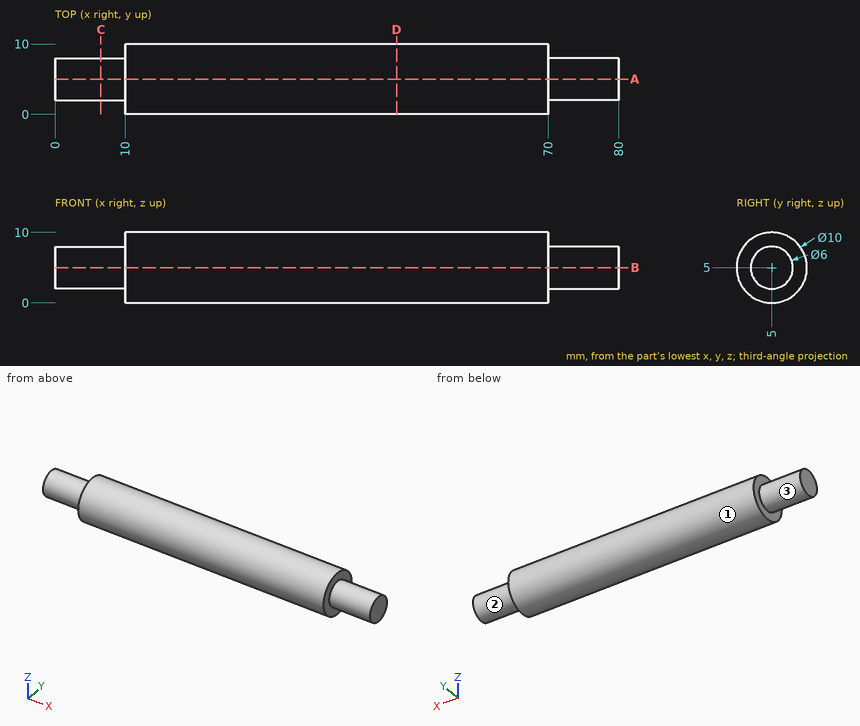
Source: three-view drawing plus pictorial views. Frame: mm from the lowest corner of the part. A direction names the side the tool comes from. Coordinates: 2 decimals unless noted, no trailing zeros. Order: outer loops, then holes, each group sorted by start corner. A loop starts at its lowest first (then second) coordinate and runs counter-clockwise, first axis right, second up. Notation, with made-up numbers: M 40.25,-10 L 61.25,-10 A33 cw 61.25,29 Z; hole C 57.25,1 d9. An arc over 180 degrees is marked long. Answer in a Markdown table with one row per item.
(1) Contact query for flat-ended pins moving along their axis: pin 1 Ø3 at (y, z) = (7.5, 7.5) entering from -X; pin 2 Ø6 at (x, z) = (14, 9) entering from +Y; pin 3 Ø1.5 at (x, z) = (35, 2) entering from +Y; pin 4 Ø3 at (y, z) = (8.5, 2) entering from +X. Output: stop coordinate, or through.
Numbers:
| item | result |
|---|---|
| pin 1 | stops at x = 0 |
| pin 2 | stops at y = 9.9 |
| pin 3 | stops at y = 9.47 |
| pin 4 | stops at x = 70 |
(2) Section query C-C, the plane x = 6.5. Output: boundary loops of the cut face in (y, z), plus the area to 3 significant figures.
Numbers:
| item | result |
|---|---|
| outline | C 5,5 d6 |
| area | 28.3 mm^2 |
(3) Access query for the marked faces 1, 2 and 3. Directions: +Z, -Z, +X, -X, +Y, -Y. A direction counts if a zero-diameter tool reaches every point of the face in a straight line with its end or side. Return the directions, or none.
Numbers:
| item | result |
|---|---|
| face 1 | +X, -X |
| face 2 | +X |
| face 3 | -X |
(4) Section query D-D, the plane x = 48.5. Output: boundary loops of the cut face in (y, z).
Numbers:
| item | result |
|---|---|
| outline | C 5,5 d10 |
(5) Section query A-A, the plane y = 5. Output: boundary loops of the cut face in (x, z).
Numbers:
| item | result |
|---|---|
| outline | M 0,2 L 10,2 L 10,0 L 70,0 L 70,2 L 80,2 L 80,8 L 70,8 L 70,10 L 10,10 L 10,8 L 0,8 Z |
(6) Material intervals for line 1 (X direction, y = 4.75, z = 0.75); line 2 (Y direction, x = 51, z = 1); line 3 (Z direction, x = 5.5, y = 4.75), sorted ascending. Write a range as [from, to].
Numbers:
| item | result |
|---|---|
| line 1 | x = [10, 70] |
| line 2 | y = [2, 8] |
| line 3 | z = [2.01, 7.99] |
